For this review, take the finished solid that the model builds, in its own axes (mm). Face numbers are marked on the shaded views. A direction names the side the tool comes from. Round coordinates to 2 decimals unless told otherwise and drop trailing zeros. Order: outer loops, then holes, each group sorted by start corner. A loop starts at its lowest first (then second) coordinate and runs counter-clockwise, first axis right, second up.
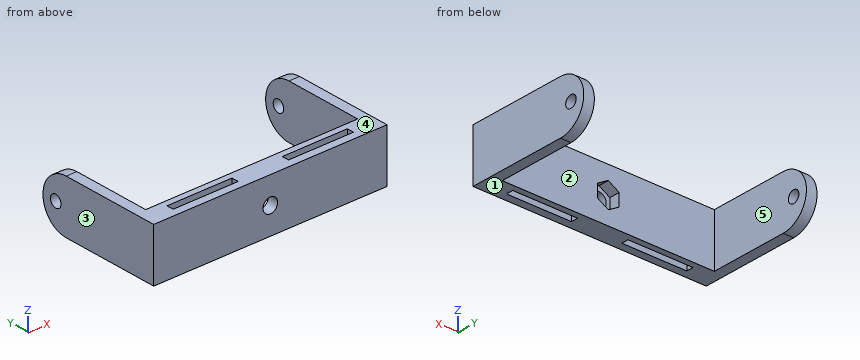
```python
from build123d import *

# Parameters (mm, degrees)
SKETCH005_W             = 80
SKETCH005_H             = 20
SKETCH005_R             = 2.75
PAD010_DEPTH            = 8
POCKET009_DEPTH         = 4
SKETCH011_W             = 24.5
SKETCH011_H             = 2.666667
POCKET010_DEPTH         = 185.699521
SKETCH017_R             = 2.25
PAD011_DEPTH            = 4
BODY002_PLACEMENT_ANGLE = 180


with BuildPart() as part:
    # Sketch005 → Pad010 (new body)
    with BuildSketch(Plane.XZ):
        Rectangle(SKETCH005_W, SKETCH005_H)
        Circle(SKETCH005_R, mode=Mode.SUBTRACT)
    extrude(amount=PAD010_DEPTH)

    # Sketch007 → Pocket009 (cut)
    with BuildSketch(Plane.XZ.offset(8)):
        Polygon((4.113621, 2.375), (0, 4.75), (-4.113621, 2.375), (-4.113621, -2.375), (0, -4.75), (4.113621, -2.375), align=None)
    extrude(amount=-POCKET009_DEPTH, mode=Mode.SUBTRACT)

    # Sketch011 → Pocket010 (cut, through all)
    with BuildSketch(Plane(origin=(0, 0, 10), x_dir=(-1, 0, 0), z_dir=(0, 0, 1))):
        with Locations((-21.75, 4.333334)):
            Rectangle(SKETCH011_W, SKETCH011_H)
    pocket010 = extrude(amount=-POCKET010_DEPTH, mode=Mode.SUBTRACT)

    # Sketch017 (on Face4 of Pad010) → Pad011 (join)
    with BuildSketch(Plane(origin=(-40, 0, 0), x_dir=(0, 0, -1), z_dir=(-1, 0, 0))):
        with BuildLine():
            Line((-10, 0), (10, 0))
            Line((10, 0), (10, 37.5))
            ThreePointArc((10, 37.5), (0, 47.5), (-10, 37.5))
            Line((-10, 37.5), (-10, 0))
        make_face()
        with Locations((0, 42)):
            Circle(SKETCH017_R, mode=Mode.SUBTRACT)
    pad011 = extrude(amount=PAD011_DEPTH)

    # Mirrored007: Pad011 across YZ
    add(pad011.mirror(Plane.YZ))

    # Mirrored008: Pocket010 across YZ
    add(pocket010.mirror(Plane.YZ), mode=Mode.SUBTRACT)


with BuildPart() as part_1:
    # Body002 placement: moved
    add(part.part.moved(Location((0, 2, 9))).rotate(Axis((0, 2, 9), (1, 0, 0)), BODY002_PLACEMENT_ANGLE))


solid = part_1.part
```
Q1. Clearance check with flat-ended pins moving along their axes: pin 1 (2.5 mm diameter, centred on x = -0.5, z = 7.5, fed in from +Y); pin 2 (6 mm diameter, centred on x = 7, z = 12, fed in from +Y); pin 3 (2.5 mm diameter, centred on y = 44, z = 9, fed in from -X). State where each tip first meets the part, or that it passes through.
Q2. Take a section at C-C, the plane x = -24.5. State the section outline as (y, z) points, plus the area to 3 significant figures.
Q3. Mouldability with a two-part tool opening along X and no side actions: class the marked faces 1, 2 and 3 as +X half, -X half, draft (parallel to the pull), parting line (faces both ways), or undercut.
Q4. Wall thickness on line 1 (Y direction, x = -42.25, z = 9); line 2 (X direction, y = 32, z = 15.5); line 3 (Y direction, x = 28, z = 8.5): over which ranges is each line inside the solid? List them lowest first.
Q5. Tool access review of the marked faces 4 and 5: name each direction out of +Z, -Z, +X, -X, +Y, -Y from which nothing blocks a thin tool from reaching the whole face with its end or side.
Q6. Take a section at D-D, the plane y = 44. State the section outline as (x, z) points, plus the area to 3 significant figures.
Q7. Take a section at B-B, the plane z = 9. Count the separate pieces of the cut face and the enclosed holes in it, plus the area to 3 significant figures.
Q8. Take a section at A-A, the plane y = 37.5. State the section outline as (x, z) points.
Working result:
1. pin 1: stops at y = 6
1. pin 2: stops at y = 10
1. pin 3: passes through
2. outline: (2, -1) - (5, -1) - (5, 19) - (2, 19) - close; (7.67, -1) - (10, -1) - (10, 19) - (7.67, 19) - close
2. area: 107 mm2
3. face 1: draft
3. face 2: undercut
3. face 3: -X half
4. line 1: y = 2 to 41.75, 46.25 to 49.5
4. line 2: x = -44 to -40, 40 to 44
4. line 3: y = 2 to 5, 7.67 to 10
5. face 4: +Z, +X, -X, +Y, -Y
5. face 5: +Z, -Z, +Y
6. outline: (-44, 0.07) - (-40, 0.07) - (-40, 6.75) - (-44, 6.75) - close; (-44, 11.25) - (-40, 11.25) - (-40, 17.93) - (-44, 17.93) - close; (40, 0.07) - (44, 0.07) - (44, 6.75) - (40, 6.75) - close; (40, 11.25) - (44, 11.25) - (44, 17.93) - (40, 17.93) - close
6. area: 107 mm2
7. separate pieces: 4
7. enclosed holes: 2
7. area: 798 mm2
8. outline: (-44, -1) - (-40, -1) - (-40, 19) - (-44, 19) - close; (40, -1) - (44, -1) - (44, 19) - (40, 19) - close
